from build123d import *

# Parameters (mm, degrees)
F2_R     = 4.7625
F3_DEPTH = 9.525
F5_R     = 1.5875
F6_DEPTH = 20.32


with BuildPart() as f1:
    # F0 (on Front) → F1 (revolve)
    with BuildSketch(Plane.XZ):
        Polygon((7.453438, 16.332791), (0, 16.332791), (0, -21.767209), (19.520697, -7.259378), (19.520697, 0), (7.453438, 0), align=None)
    revolve(axis=Axis((0, 0, -2.717209), (0, 0, -1)))

    # F2 (on face) → F3 (cut)
    with BuildSketch(Plane.XY.offset(16.332791)):
        Circle(F2_R)
    extrude(amount=-F3_DEPTH, mode=Mode.SUBTRACT)

    # F5 (on offset) → F6 (cut)
    with BuildSketch(Plane.XY.offset(-22.225)):
        Circle(F5_R)
    extrude(amount=F6_DEPTH, mode=Mode.SUBTRACT)


solid = f1.part
Build history of the part. All positions in model axes, mm. A direction names the side the tool comes from. Coordinates: 2 decimals unless noted, no trailing zeros. Order: outer loops, then holes, each group sorted by start corner. A loop starts at its lowest first (then second) coordinate and runs counter-clockwise, first axis right, second up. Notation, with made-up numbers: (61, 57) - (110, 57) arc R31 ccw to (110, 87) - close; hole circle Ø1 at (-6.75, -26.5). An arc over 180 degrees is marked (long way). Put each result on its own line as item: value.
1. Saw through at A-A (y = 0). Write the cut outline in (x, z) (1 decimal), and give its area (3 significant figures).
Answer sheet:
outline: (-19.5, -7.3) - (-1.6, -20.6) - (-1.6, -1.9) - (1.6, -1.9) - (1.6, -20.6) - (19.5, -7.3) - (19.5, 0) - (7.5, 0) - (7.5, 16.3) - (4.8, 16.3) - (4.8, 6.8) - (-4.8, 6.8) - (-4.8, 16.3) - (-7.5, 16.3) - (-7.5, 0) - (-19.5, 0) - close
area: 658 mm^2
2. Saw through at C-C (z = 13). Write the cut outline in (x, y) (1 decimal), and give its area (3 significant figures).
Answer sheet:
outline: circle Ø14.9 at (0, 0); hole circle Ø9.5 at (0, 0)
area: 103 mm^2
3. Probe line 1 along X through (y, z) = (0, -16); line 2 along Y through (x, z) = (0, 9.5); line 3 along Y through (x, z) = (0, -15.5). List the from-to ranges inside material, lowest first. Write a range as [from, to].
Answer sheet:
line 1: x = [-7.76, -1.59], [1.59, 7.76]
line 2: y = [-7.45, -4.76], [4.76, 7.45]
line 3: y = [-8.43, -1.59], [1.59, 8.43]
4. Tool access for faces 5 (the face through (8, 0, 0)), 6 (the face through (-1.019, 4.59, -18.273)): list every direction of +Z, -Z, +X, -X, +Y, -Y with a clear straight run to the whole face (end or side of a thin tool).
Answer sheet:
face 5: +Z
face 6: -Z
5. Drop flat-ended pins along their axis: P1, Ø1.9, axis at x = 0, y = 0, coming from the -Z side (3 decimals); P2, Ø3, axis at y = 2.5, z = -7, coming from the -X side; P3, Ø12, axis at x = -13.5, z = -15, coming from the +Y side. Give the stop position or say it passes through.
Answer sheet:
P1: stops at z = -1.905
P2: stops at x = -19.5
P3: stops at y = 12.23
6. Saw through at D-D (z = -6.5). Write the cut outline in (x, y) (1 decimal), and give its area (3 significant figures).
Answer sheet:
outline: circle Ø39 at (0, 0); hole circle Ø3.2 at (0, 0)
area: 1,190 mm^2
7. Pull direction Y, two halves, no side cores. Call faces 1 (the face through (-4.232, 19.057, -3.579)), 2 (the face through (5, 0, 16.333)), 3 (the face through (-0.34, -1.55, -11.38)), 4 (the face through (0, 0, -1.905)): pulls with the +Y half, pulls with the -Y half, needs draft (parallel to the pull), parting line crosses it, or undercut.
Answer sheet:
face 1: parting line crosses it
face 2: needs draft
face 3: undercut
face 4: undercut
